Verification items for this drawing (mm, ordinates from the low corner). Round coordinates to 2 decimals unless told otherwise and drop trailing zeros. Order: outer loops, then holes, each group sorted by start corner. A loop starts at its lowest first (then second) coordinate and runs counter-clockwise, first axis right, second up. Notation, with made-up numbers: (45.5, 72) -> (67.5, 72) arc R24 cw to (67.5, 94) -> close; hole circle Ø2 at (-33.75, -5.75). An arc over 180 degrees is marked (long way). Answer in a Markdown table with one row per item. Add a question column.
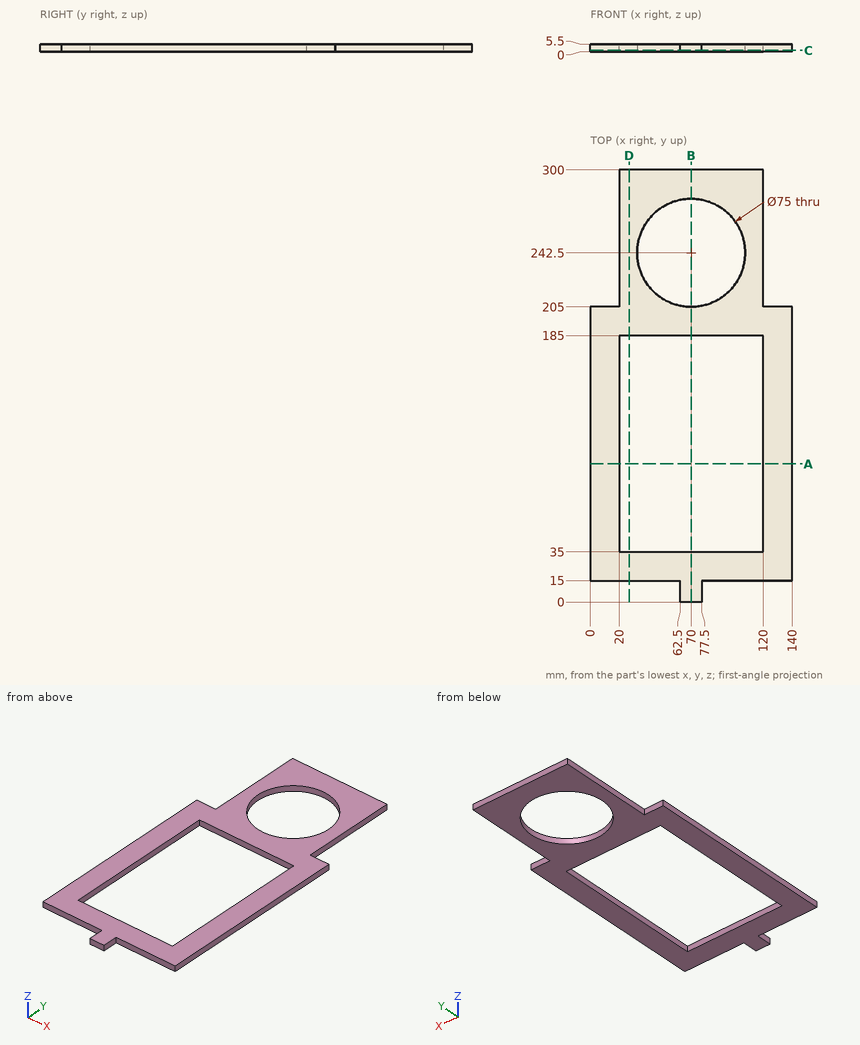
1) Thickness scan on L1, parallel to Y at x = 70, z = 3.6; L2, parallel to Y at x = 68, z = 4.6; L3, parallel to X at y = 242.5, z = 2.75. Record the ranges inside material, lowest first. Write a range as [from, to].
2) Cross-section at B-B, the plane x = 70. Record the boundary of the cut face in (y, z).
3) Cross-section at C-C, the plane z = 1. Record the boundary of the cut face in (x, y).
4) Cross-section at D-D, the plane x = 27. Record the boundary of the cut face in (y, z), and give its area (4 significant figures).
5) Cross-section at A-A, the plane y = 96. Record the boundary of the cut face in (x, z).
6) Depth check by flat-ended pin: P1, Ø3, axis at x = 104.5, z = 2, coming from the -Y side; P2, Ø3, axis at y = 215.5, z = 1, coming from the +X side; P3, Ø1, axis at x = 106.5, y = 197.5, coming from the -Z side; P4, Ø3, axis at y = 258, z = 3, coming from the -X side. Enter the tip coordinate at first touch or a pass-through.
Results below:
| question | item | result |
|---|---|---|
| 1 | L1 | [0, 35], [185, 205], [280, 300] |
| 1 | L2 | [0, 35], [185, 205.05], [279.95, 300] |
| 1 | L3 | [20, 32.5], [107.5, 120] |
| 2 | outline | (0, 0) -> (35, 0) -> (35, 5.5) -> (0, 5.5) -> close; (185, 0) -> (205, 0) -> (205, 5.5) -> (185, 5.5) -> close; (280, 0) -> (300, 0) -> (300, 5.5) -> (280, 5.5) -> close |
| 3 | outline | (0, 15) -> (62.5, 15) -> (62.5, 0) -> (77.5, 0) -> (77.5, 15) -> (140, 15) -> (140, 205) -> (120, 205) -> (120, 300) -> (20, 300) -> (20, 205) -> (0, 205) -> close; hole (20, 35) -> (120, 35) -> (120, 185) -> (20, 185) -> close; hole circle Ø75 at (70, 242.5) |
| 4 | outline | (15, 0) -> (35, 0) -> (35, 5.5) -> (15, 5.5) -> close; (185, 0) -> (300, 0) -> (300, 5.5) -> (185, 5.5) -> close |
| 4 | area | 742.5 mm² |
| 5 | outline | (0, 0) -> (20, 0) -> (20, 5.5) -> (0, 5.5) -> close; (120, 0) -> (140, 0) -> (140, 5.5) -> (120, 5.5) -> close |
| 6 | P1 | y = 15 |
| 6 | P2 | x = 120 |
| 6 | P3 | z = 0 |
| 6 | P4 | x = 20 |
